Design review of the part built by this model. Coordinates are the model's own, in mm. A direction names the side the tool comes from. Give positions to 0.01 mm unless a question says otherwise; leave off trailing zeros. Order: outer loops, then holes, each group sorted by start corner. A loop starts at its lowest first (then second) coordinate and runs counter-clockwise, first axis right, second up. Notation, with made-up numbers: (41, -17.5) -> (48, -17.5) arc R19 ccw to (48, 7.5) -> close; hole circle Ø10 at (-23, 75.25). An arc over 180 degrees is marked (long way). One line per item, written item: value.
from build123d import *

# Parameters (mm, degrees)
SKETCH1_W             = 140
SKETCH1_H             = 140
BOSS_EXTRUDE1_DEPTH   = 3
M3X0_5_TAPPED_HOLE1_D = 3
SKETCH8_R             = 3
CUT_EXTRUDE2_DEPTH    = 2


with BuildPart() as part:
    # Sketch1 → Boss-Extrude1 (new body)
    with BuildSketch(Plane.XY):
        with Locations((70, 70)):
            Rectangle(SKETCH1_W, SKETCH1_H)
    extrude(amount=BOSS_EXTRUDE1_DEPTH)

    # M3x0.5 Tapped Hole1 (through all)
    with Locations(Plane(origin=(0, 0, 0), x_dir=(-1, 0, 0), z_dir=(0, 0, -1))):
        with Locations((-130, 92), (-130, 48), (-10, 92), (-10, 48)):
            Hole(M3X0_5_TAPPED_HOLE1_D / 2)

    # Sketch8 → Cut-Extrude2 (cut)
    with BuildSketch(Plane(origin=(0, 0, 0), x_dir=(-1, 0, 0), z_dir=(0, 0, -1))):
        with Locations((-70, 70)):
            Circle(SKETCH8_R)
    extrude(amount=-CUT_EXTRUDE2_DEPTH, mode=Mode.SUBTRACT)


solid = part.part
Item 1: Machinability: for faces 1 (the flat face through (70, 70, 2)), 2 (the flat face through (69, 55, 0)), which of the approach directions +Z, -Z, +X, -X, +Y, -Y give a long, thin tool a straight path to every point of the face, cutting with its end or side? Answer none if there is none.
Returned:
face 1: -Z
face 2: -Z, +X, -X, +Y, -Y
Item 2: Add section A-A on y = 70. Give the boundary of the cut face in (x, z), plus the area to 3 significant figures.
Returned:
outline: (0, 0) -> (67, 0) -> (67, 2) -> (73, 2) -> (73, 0) -> (140, 0) -> (140, 3) -> (0, 3) -> close
area: 408 mm²
Item 3: To check wall thickness, follow line 1 along Y through (x, z) = (130, 1.5); line 2 along X through (y, z) = (92, 0.7); line 3 along Y through (x, z) = (70, 1.1). State the ranges of each line that lie inside material, in increasing order. Write a range as from..to.
Returned:
line 1: 0..46.5, 49.5..90.5, 93.5..140
line 2: 0..8.5, 11.5..128.5, 131.5..140
line 3: 0..67, 73..140
Item 4: Draft analysis for pull direction Y (two halves, no side actions). For faces 3 (the cylindrical face through (72.4, 68.2, 1)), 4 (the cylindrical face through (128.89, 93.01, 1.52)), 5 (the flat face through (69, 0, 1)), 6 (the flat face through (140, 69, 1)), state which applies: pulls with the +Y half, pulls with the -Y half, needs draft (parallel to the pull), parting line crosses it, or undercut.
Returned:
face 3: undercut
face 4: undercut
face 5: pulls with the -Y half
face 6: needs draft
